CAD build for the part. Positions are in the model's coordinates, mm. A direction names the side the tool comes from. Round coordinates to 2 decimals unless told otherwise and drop trailing zeros. Order: outer loops, then holes, each group sorted by start corner. A loop starts at its lowest first (then second) coordinate and runs counter-clockwise, first axis right, second up. Notation, with made-up numbers: M 24,69 L 52,69 A13 ccw 52,85 Z; hole C -10.5,45.25 d5. An arc over 180 degrees is marked long. Answer as a JSON object with one key per item and string values.
```python
from build123d import *

# Parameters (mm, degrees)
SKETCH1_W                      = 20
SKETCH1_H                      = 20
BOSS_EXTRUDE1_DEPTH            = 2
BOSS_EXTRUDE3_DEPTH            = 1.5
TAP_DRILL_FOR_M2_2_HELICOIL1_D = 6.5


with BuildPart() as part:
    # Sketch1 → Boss-Extrude1 (new body)
    with BuildSketch(Plane(origin=(0, 0, 0), x_dir=(1, 0, 0), z_dir=(0, 1, 0))):
        Rectangle(SKETCH1_W, SKETCH1_H)
    extrude(amount=BOSS_EXTRUDE1_DEPTH)

    # Sketch3 → Boss-Extrude3 (add)
    with BuildSketch(Plane(origin=(0, 2, 0), x_dir=(1, 0, 0), z_dir=(0, 1, 0))):
        Polygon((-2.875, 8.25), (2.875, 8.25), (2.875, 2.867474963), (8.25, 2.867474963), (8.25, -2.882525037), (2.875, -2.875), (2.875, -8.25), (-2.875, -8.25), (-2.875, -2.875), (-8.25, -2.875), (-8.25, 2.875), (-2.875, 2.875), align=None)
    extrude(amount=BOSS_EXTRUDE3_DEPTH)

    # Tap Drill for M2.2 Helicoil1 (through all)
    with Locations(Plane.ZX.offset(3.5)):
        with Locations((0, 0)):
            Hole(TAP_DRILL_FOR_M2_2_HELICOIL1_D / 2)


solid = part.part
```
Item 1: Wall check: line 1 along X through (y, z) = (1.05, 0); line 2 along Y through (x, z) = (7.5, -7.5); line 3 along X through (y, z) = (3.2, 5.5) (3 decimals). Give the ranges that are in metal, low to high. Write a range as [from, to].
Worked answers:
{"line 1": "x = [-10, -3.25], [3.25, 10]", "line 2": "y = [0, 2]", "line 3": "x = [-2.875, 2.875]"}
Item 2: Saw through at A-A on z = 0. List the corners of the cut face in (x, y), and give its area (3 significant figures).
Worked answers:
{"outline": "M -10,0 L -3.25,0 L -3.25,3.5 L -8.25,3.5 L -8.25,2 L -10,2 Z; M 3.25,0 L 10,0 L 10,2 L 8.25,2 L 8.25,3.5 L 3.25,3.5 Z", "area": "42.0 mm2"}
Item 3: Saw through at C-C on y = 1.6. List the corners of the cut face in (x, z).
Worked answers:
{"outline": "M -10,-10 L 10,-10 L 10,10 L -10,10 Z; hole C 0,0 d6.5"}
Item 4: 3-axis set-ups, long thin cutter, end or side, ignore diameter. For faces 1 (the flat face through (2.875, 3, 6)), 2 (the flat face through (-2.875, 3, -6)), 3 (the flat face through (-2.875, 3, 6)): which of +Z, -Z, +X, -X, +Y, -Y reach the whole face in a straight line?
Worked answers:
{"face 1": "+Z, +X, +Y", "face 2": "-Z, -X, +Y", "face 3": "+Z, -X, +Y"}
Item 5: Saw through at D-D on z = -7.75. List the corners of the cut face in (x, y) (3 decimals), and give its area (3 significant figures).
Worked answers:
{"outline": "M -10,0 L 10,0 L 10,2 L 2.875,2 L 2.875,3.5 L -2.875,3.5 L -2.875,2 L -10,2 Z", "area": "48.6 mm2"}
Item 6: Drop flat-ended pins along their axis: pin 1 Ø1.2 at (y, z) = (3, -5.5) entering from +X (3 decimals); pin 2 Ø1.2 at (x, y) = (-0.5, 3) entering from +Z; pin 3 Ø0.8 at (x, y) = (6.5, 3) entering from -Z. Give the stop position or say it passes through.
Worked answers:
{"pin 1": "stops at x = 2.875", "pin 2": "stops at z = 8.25", "pin 3": "stops at z = -2.87"}
Item 7: Saw through at B-B on x = 0. List the corners of the cut face in (y, z).
Worked answers:
{"outline": "M 0,-10 L 2,-10 L 2,-8.25 L 3.5,-8.25 L 3.5,-3.25 L 0,-3.25 Z; M 0,3.25 L 3.5,3.25 L 3.5,8.25 L 2,8.25 L 2,10 L 0,10 Z"}
Item 8: Two-plate mould, pull along Z, no slides. Class faces 4 (the flat face through (0, 1, -10)), 5 (the cylindrical face through (-1.978, 1.726, 2.579)), 6 (the flat face through (-8.25, 3, 0)), 7 (the flat face through (0, 1, 10)): released by +Z, released by -Z, zero draft, split by the parting line, or undercut.
Worked answers:
{"face 4": "released by -Z", "face 5": "undercut", "face 6": "zero draft", "face 7": "released by +Z"}
